Read the model definition and answer for the solid it produces. Units are mm, in the model's axes. Face numbers are marked on the shaded views. A direction names the side the tool comes from. Coordinates: 2 decimals unless noted, no trailing zeros. Order: outer loops, then holes, each group sorted by start corner. A loop starts at its lowest first (then second) coordinate and runs counter-clockwise, first axis right, second up. Notation, with made-up numbers: (-37, 71.5) -> (14, 71.5) arc R18 ccw to (14, 97.5) -> close; hole circle Ø3 at (10.25, 6.5). An arc over 180 degrees is marked (long way). Use CSV: the item, a comma, the result in double quotes.
```python
from build123d import *

# Parameters (mm, degrees)
SKETCH_1_R      = 20
SKETCH_1_R_2    = 5
SKETCH_1_W      = 5
SKETCH_1_H      = 2.6
SKETCH_1_W_2    = 2.6
SKETCH_1_H_2    = 5
SKETCH_1_W_3    = 2.8
SKETCH_1_W_4    = 2.941603816
SKETCH_1_H_3    = 2.897870759
SKETCH_1_H_4    = 2.841528046
EXTRUDE_1_DEPTH = 10


with BuildPart() as part:
    # Эскиз1 → Бобышка-Вытянуть1 (new body)
    with BuildSketch(Plane(origin=(0, 0, 0), x_dir=(1, 0, 0), z_dir=(0, 1, 0))):
        with Locations(Location((0, 0, 0), (0, 0, 270))):
            Circle(SKETCH_1_R)
        with Locations(Location((0, 0, 0), (0, 0, 270))):
            Circle(SKETCH_1_R_2, mode=Mode.SUBTRACT)
        with Locations((0, -14.7)):
            Rectangle(SKETCH_1_W, SKETCH_1_H, mode=Mode.SUBTRACT)
        with Locations((-14.7, 0)):
            Rectangle(SKETCH_1_W_2, SKETCH_1_H_2, mode=Mode.SUBTRACT)
        with Locations((14.7, 0)):
            Rectangle(SKETCH_1_W_2, SKETCH_1_H_2, mode=Mode.SUBTRACT)
        with Locations((0, 14.7)):
            Rectangle(SKETCH_1_W, SKETCH_1_H, mode=Mode.SUBTRACT)
        with Locations((8.896405813, 8.788682263)):
            Rectangle(SKETCH_1_W_3, SKETCH_1_H_2, mode=Mode.SUBTRACT)
        with Locations((-8.402919516, -8.301171423)):
            Rectangle(SKETCH_1_W_4, SKETCH_1_H_2, mode=Mode.SUBTRACT)
        with Locations((-8.314700298, 8.958870068)):
            Rectangle(SKETCH_1_W, SKETCH_1_H_3, mode=Mode.SUBTRACT)
        with Locations((8.878230894, -8.443187871)):
            Rectangle(SKETCH_1_W, SKETCH_1_H_4, mode=Mode.SUBTRACT)
    extrude(amount=EXTRUDE_1_DEPTH)


solid = part.part
```
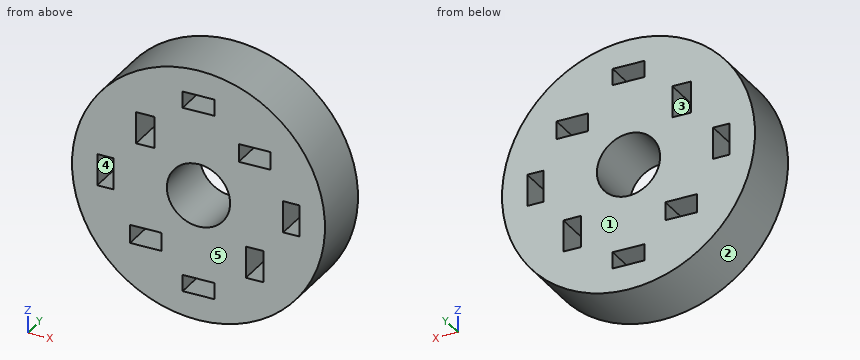
Item 1: Find section C-C, the plane y = 3.5. Give the number of separate pieces and of enclosed holes in the cut face, then the cut area to 3 significant figures.
Return value:
separate pieces,"1"
enclosed holes,"9"
area,"1,070 mm^2"
Item 2: Each of these flat-tipped pins is pushed along its axis until it touches: P1, Ø1.5, axis at x = -1, y = 7, coming from the +Z side; P2, Ø0.8, axis at x = 15, y = 5.5, coming from the -Z side; P3, Ø2, axis at x = -4.5, y = 5, coming from the -Z side; P4, Ø2, axis at x = 0, z = 2, coming from the -Y side. Where does it stop, or does it pass through?
Return value:
P1,"stops at z = 20"
P2,"stops at z = -13.67"
P3,"stops at z = -19.69"
P4,"passes through"
Item 3: The mould has two halves that part along Z. Classify the marked faces 1, 2 and 3: +Z half, -Z half, draft (parallel to the pull), parting line (faces both ways), or undercut.
Return value:
face 1,"draft"
face 2,"parting line"
face 3,"undercut"
Item 4: A tool of negligible diameter and unlimited length cuts with its end or side. For the marked faces 4 and 5, from which of +Z, -Z, +X, -X, +Y, -Y can it reach the whole face along a straight path? Write none if from no direction.
Return value:
face 4,"+Y, -Y"
face 5,"+Z, -Z, +X, -X, -Y"
Item 5: Find section B-B, the plane x = 0. Give the vertices of the cut face in (y, z), then the cut area to 3 significant figures.
Return value:
outline,"(0, -20) -> (10, -20) -> (10, -16) -> (0, -16) -> close; (0, -13.4) -> (10, -13.4) -> (10, -5) -> (0, -5) -> close; (0, 5) -> (10, 5) -> (10, 13.4) -> (0, 13.4) -> close; (0, 16) -> (10, 16) -> (10, 20) -> (0, 20) -> close"
area,"248 mm^2"
Item 6: Straight lines are drawn through the part: line 1 along X through (y, z) = (3.5, 0); line 2 along Z through (x, y) = (9, 4); line 3 along Z through (x, y) = (9.5, 7). For each, find the intervals that lie inside material, in ascending order.
Return value:
line 1,"x = -20 to -16, -13.4 to -5, 5 to 13.4, 16 to 20"
line 2,"z = -17.86 to -11.29, -6.29 to 7.02, 9.86 to 17.86"
line 3,"z = -17.6 to -11.29, -6.29 to 7.02, 9.86 to 17.6"
Item 7: Find section D-D, the plane x = 15. Give the vertices of the cut face in (y, z).
Return value:
outline,"(0, -13.23) -> (10, -13.23) -> (10, -2.5) -> (0, -2.5) -> close; (0, 2.5) -> (10, 2.5) -> (10, 13.23) -> (0, 13.23) -> close"
Item 8: Find section A-A, the plane z = 0. Give the vertices of the cut face in (x, y), then the cut area to 3 significant figures.
Return value:
outline,"(-20, 0) -> (-16, 0) -> (-16, 10) -> (-20, 10) -> close; (-13.4, 0) -> (-5, 0) -> (-5, 10) -> (-13.4, 10) -> close; (5, 0) -> (13.4, 0) -> (13.4, 10) -> (5, 10) -> close; (16, 0) -> (20, 0) -> (20, 10) -> (16, 10) -> close"
area,"248 mm^2"
